from build123d import *

# Parameters (mm, degrees)
SKETCH_1_W          = 126
SKETCH_1_H          = 80
EXTRUDE_1_DEPTH     = 25
SKETCH_2_W          = 76
SKETCH_2_H          = 21
CUT_EXTRUDE_1_DEPTH = 7
SKETCH_3_W          = 76
SKETCH_3_H          = 21
CUT_EXTRUDE_2_DEPTH = 7
SKETCH_4_R          = 3.5
CUT_EXTRUDE_3_DEPTH = 7
SKETCH_5_R          = 1.5
CUT_EXTRUDE_5_DEPTH = 23
SKETCH_6_R          = 1.5
CUT_EXTRUDE_6_DEPTH = 23


with BuildPart() as part:
    # 草图1 → 凸台-拉伸1 (new body)
    with BuildSketch(Plane(origin=(0, 0, 0), x_dir=(1, 0, 0), z_dir=(0, 1, 0))):
        with Locations((63, -40)):
            Rectangle(SKETCH_1_W, SKETCH_1_H)
    extrude(amount=EXTRUDE_1_DEPTH)

    # 草图2 → 切除-拉伸1 (cut)
    with BuildSketch(Plane(origin=(126, 0, 0), x_dir=(0, 0, -1), z_dir=(1, 0, 0))):
        with Locations((-40, 12.5)):
            Rectangle(SKETCH_2_W, SKETCH_2_H)
    extrude(amount=-CUT_EXTRUDE_1_DEPTH, mode=Mode.SUBTRACT)

    # 草图3 → 切除-拉伸2 (cut)
    with BuildSketch(Plane.ZY):
        with Locations((40, 12.5)):
            Rectangle(SKETCH_3_W, SKETCH_3_H)
    extrude(amount=-CUT_EXTRUDE_2_DEPTH, mode=Mode.SUBTRACT)

    # 草图4 → 切除-拉伸3 (cut)
    with BuildSketch(Plane(origin=(119, 0, 0), x_dir=(0, 0, -1), z_dir=(1, 0, 0))):
        with Locations((-11.90518779, 14.841361907)):
            Circle(SKETCH_4_R)
    extrude(amount=-CUT_EXTRUDE_3_DEPTH, mode=Mode.SUBTRACT)

    # 草图5 → 切除-拉伸5 (cut)
    with BuildSketch(Plane(origin=(0, 2, 0), x_dir=(1, 0, 0), z_dir=(0, 1, 0))):
        with Locations(Location((122.5, -17.5, 0), (0, 0, 270))):
            Circle(SKETCH_5_R)
        with Locations(Location((122.5, -32.5, 0), (0, 0, 270))):
            Circle(SKETCH_5_R)
        with Locations(Location((122.5, -47.5, 0), (0, 0, 270))):
            Circle(SKETCH_5_R)
        with Locations(Location((122.5, -62.5, 0), (0, 0, 270))):
            Circle(SKETCH_5_R)
    extrude(amount=-CUT_EXTRUDE_5_DEPTH, mode=Mode.SUBTRACT)

    # 草图6 → 切除-拉伸6 (cut)
    with BuildSketch(Plane(origin=(0, 2, 0), x_dir=(1, 0, 0), z_dir=(0, 1, 0))):
        with Locations(Location((3.5, -17.5, 0), (0, 0, 270))):
            Circle(SKETCH_6_R)
        with Locations(Location((3.5, -32.5, 0), (0, 0, 270))):
            Circle(SKETCH_6_R)
        with Locations(Location((3.5, -47.5, 0), (0, 0, 270))):
            Circle(SKETCH_6_R)
        with Locations(Location((3.5, -62.5, 0), (0, 0, 270))):
            Circle(SKETCH_6_R)
    extrude(amount=-CUT_EXTRUDE_6_DEPTH, mode=Mode.SUBTRACT)


solid = part.part
The listing builds one solid part. Answer for the finished solid, in the listing's coordinates (mm). A direction names the side the tool comes from. Coordinates: 2 decimals unless noted, no trailing zeros. Loops run counter-clockwise (first coordinate to the right, second up) from the corner with the lowest first, then second, coordinate; pieces in that order, holes last. Notation, with made-up numbers: M 23.25,82 L 70.25,82 A27 ccw 70.25,106 Z; hole C 24,45 d1. An arc over 180 degrees is marked long. Answer in a Markdown table with one row per item.
1) Find section D-D (z = 25). Determine the outline of the cut face in (x, y).
Answers below:
| item | result |
|---|---|
| outline | M 0,0 L 126,0 L 126,2 L 119,2 L 119,23 L 126,23 L 126,25 L 0,25 L 0,23 L 7,23 L 7,2 L 0,2 Z |
2) Which of the six approach directions +Z, -Z, +X, -X, +Y, -Y give full straight-line access (tool end or side, diameter ignored) to faces 4 (the flat face through (3, 12, 78)), 5 (the cylindrical face through (3.57, 1.01, 46)), 6 (the flat face through (123, 12, 78)), 7 (the flat face through (126, 24, 43))?
Answers below:
| item | result |
|---|---|
| face 4 | -X |
| face 5 | -Y |
| face 6 | +X |
| face 7 | +Z, -Z, +X, +Y, -Y |
3) Determine the mould class of faces 1 (the flat face through (62, 0, 39)), 2 (the flat face through (62, 12, 80)), 3 (the cylindrical face through (123.987, 1.014, 47.305)) for opening direction Z: released by +Z, released by -Z, zero draft, split by the parting line, or undercut.
Answers below:
| item | result |
|---|---|
| face 1 | zero draft |
| face 2 | released by +Z |
| face 3 | undercut |
4) Find the intervals of material crossed by probe 1 along X at (y, z) = (0.6, 17.5); probe 2 along Z at (x, y) = (122.5, 0.75); probe 3 along X at (y, z) = (4.5, 10.5), in increasing order.
Answers below:
| item | result |
|---|---|
| probe 1 | 0 to 2, 5 to 121, 124 to 126 |
| probe 2 | 0 to 16, 19 to 31, 34 to 46, 49 to 61, 64 to 80 |
| probe 3 | 7 to 119 |
5) Given pin 1 (6 mm diameter, centred on y = 16, z = 15, fed in from -X); pin 2 (1.8 mm diameter, centred on x = 3.5, z = 32.5, fed in from -Y); pin 3 (10.5 mm diameter, centred on y = 12, z = 54.5, fed in from +X), each flat-ended and moving along its own axis, determine where each tip first touches the part or whether it passes through.
Answers below:
| item | result |
|---|---|
| pin 1 | x = 7 |
| pin 2 | y = 23 |
| pin 3 | x = 119 |
6) Find section B-B (z = 47.5). Determine the outline of the cut face in (x, y), then the cut area to 3 significant figures.
Answers below:
| item | result |
|---|---|
| outline | M 0,0 L 2,0 L 2,2 L 0,2 Z; M 0,23 L 7,23 L 7,2 L 5,2 L 5,0 L 121,0 L 121,2 L 119,2 L 119,23 L 126,23 L 126,25 L 0,25 Z; M 124,0 L 126,0 L 126,2 L 124,2 Z |
| area | 2,840 mm^2 |
7) Find section A-A (x = 122.5). Determine the outline of the cut face in (y, z), then the cut area to 3 significant figures.
Answers below:
| item | result |
|---|---|
| outline | M 0,0 L 25,0 L 25,80 L 0,80 L 0,64 L 2,64 L 2,78 L 23,78 L 23,2 L 2,2 L 2,16 L 0,16 Z; M 0,19 L 2,19 L 2,31 L 0,31 Z; M 0,34 L 2,34 L 2,46 L 0,46 Z; M 0,49 L 2,49 L 2,61 L 0,61 Z |
| area | 380 mm^2 |
8) Find section C-C (y = 19.75). Determine the outline of the cut face in (x, z).
Answers below:
| item | result |
|---|---|
| outline | M 0,0 L 126,0 L 126,2 L 119,2 L 119,78 L 126,78 L 126,80 L 0,80 L 0,78 L 7,78 L 7,2 L 0,2 Z |
